Check sheet for the drawn part. Datum: minimum x, y, z corner. Units: mm. A direction names the side the tool comes from. Round coordinates to 2 decimals unless told otherwise and drop trailing zeros. Write each loop counter-clockwise with the first axis right and the second up, starting at its lowest first coordinate (ties: lowest second). Pieces come first, ordered by that corner, then holes.
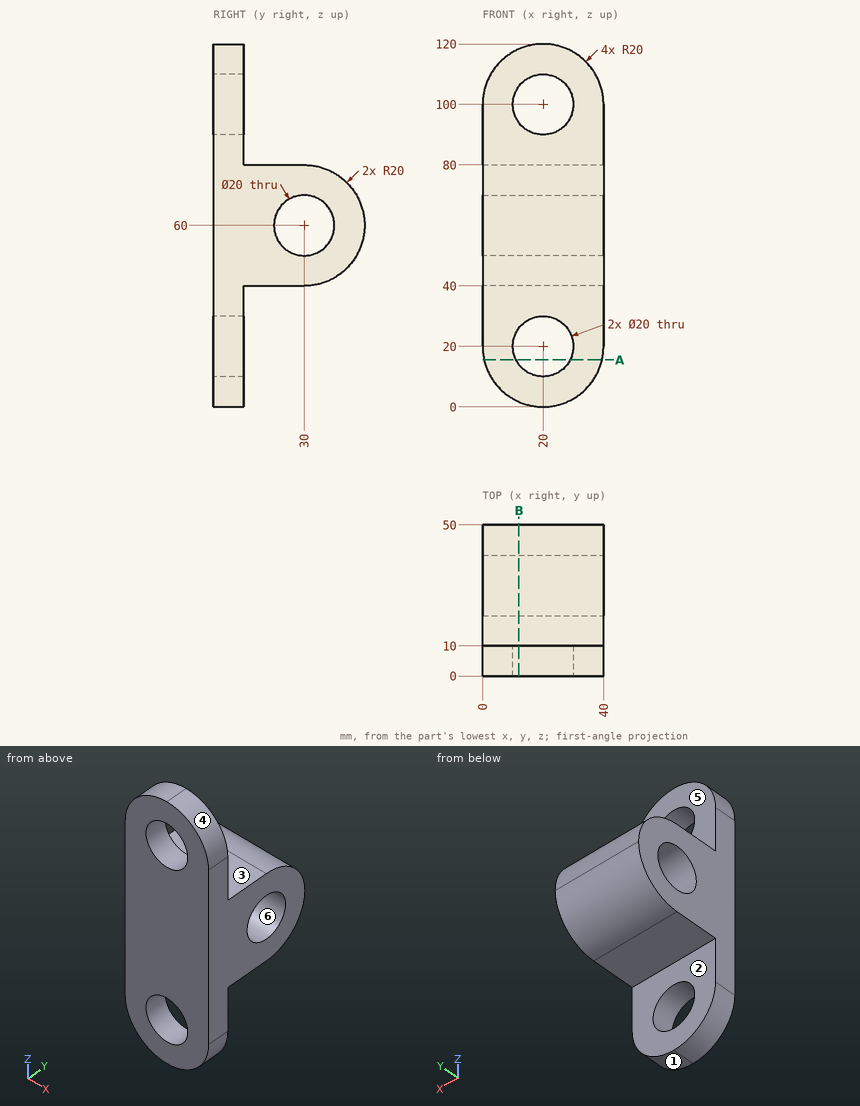
Q1. Sectioned sample at B-B (x = 12). Give the number of separate pieces and of enclosed holes in the cut face, plus the area to 3 significant figures.
Recorded:
separate pieces: 3
enclosed holes: 1
area: 2,040 mm2
Q2. Material ranges on line 1 along Z through (x, y) = (20, 4); line 2 along Y through (x, z) = (24, 60); line 3 along Z through (x, y) = (29.5, 30.5), recorded low to high.
Recorded:
line 1: z = 0 to 10, 30 to 90, 110 to 120
line 2: y = 0 to 20, 40 to 50
line 3: z = 40.01 to 50.01, 69.99 to 79.99
Q3. Tool access check on the marked faces 1, 2 and 3. Record the directions out of +Z, -Z, +X, -X, +Y, -Y that give a thin tool (end or side, any length) a straight path to the whole face; none if there is none.
Recorded:
face 1: -Z, +X, +Y, -Y
face 2: -Z, +X, -X, +Y
face 3: +Z, +X, -X, +Y
Q4. Depth check by flat-ended pin: P1, Ø12, axis at x = 29.5, z = 93.5, coming from the +Y side; P2, Ø2, axis at x = 29, z = 64, coming from the -Y side; P3, Ø10, axis at x = 18, y = 15.5, coming from the -Z side; P4, Ø16, axis at x = 25, y = 19.5, coming from the +Z side. Enter the tip coordinate at first touch or a pass-through.
Recorded:
P1: stops at y = 10
P2: stops at y = 0
P3: stops at z = 40
P4: stops at z = 80
Q5. Sectioned sample at A-A (z = 15.5). Enter the section's corners in (x, y), plus the area to 3 significant figures.
Recorded:
outline: (0.51, 0) - (11.07, 0) - (11.07, 10) - (0.51, 10) - close; (28.93, 0) - (39.49, 0) - (39.49, 10) - (28.93, 10) - close
area: 211 mm2
Q6. Release check for a two-part mould opening along Z. For the marked faces 4, 5 and 6 record: released by +Z, released by -Z, zero draft, split by the parting line, or undercut.
Recorded:
face 4: released by +Z
face 5: zero draft
face 6: undercut
